Can you work these out from the model? Positions are in its coordinate system, mm. A direction names the side the tool comes from. Round coordinates to 2 decimals unless told otherwise and drop trailing zeros. Write each loop counter-clockwise with the first axis right and the second up, starting at its lowest first coordinate (ties: lowest second). Pieces come first, ordered by that corner, then holes. Notation, with made-up numbers: M 86.25,84.5 L 93.25,84.5 A5 cw 93.25,91.5 Z; hole C 24,31.25 d6. An arc over 180 degrees is marked long. Answer in a Markdown table with one row per item. Add a question column.
(1) I'm going to push flat-ended pins straight in: pin 1 (0.8 mm diameter, centred on x = -17.5, y = -6, fed in from +Z); pin 2 (4.5 mm diameter, centred on x = -12.5, z = 10.5, fed in from -Y); pin 3 (1.5 mm diameter, centred on y = -3, z = 11.5, fed in from +X). Where does each tip first touch, or does it pass through?
(2) For faces 1 (the face through (10, -6, 5)), 2 (the face through (23, 5.2, 5)), 3 (the face through (11.343, 18.021, 3.889)), 4 (the face through (13, 6, 8)), 5 (the face through (0, 14.6, 1)), which set-ups out of +Z, -Z, +X, -X, +Y, -Y let a thin tool reach every point of the face, with its end or its side?
(3) Suppose I cut it at C-C, the plane x = 4. Write out the boundary of the cut face in (y, z).
(4) If I drill on probe 1 along Y at (x, z) = (-13, 5.25); probe 2 along X at (y, z) = (-6.5, 10.25); probe 3 along Y at (x, z) = (19, 13.25), over which ranges is the centre line in solid material (lowest first)?
(5) Suppose I cut it at D-D, the plane y = -4.5. Write out the boundary of the cut face in (x, z), then the cut area to 3 significant figures.
(6) Suppose I cut it at B-B, the plane x = -8.5. Write out the boundary of the cut face in (y, z), then the cut area to 3 significant figures.
(7) If we mould it in two halves opening along X, with no side actions, what happens to faces 6 (the face through (-22.5, -12.5, 1.5)), 7 (the face through (0, -10.4, 1)), 8 (the face through (25, 0, 2)), 9 (the face through (-22, 17, 4))? For each: released by +X, released by -X, zero draft, split by the parting line, or undercut.
(8) Suppose I cut it at A-A, the plane y = -12.5. Write out the boundary of the cut face in (x, z), then the cut area to 3 significant figures.
from build123d import *

# Parameters (mm, degrees)
SZKIC1_W                    = 50
SZKIC1_H                    = 34
DODANIE_WYCI_GNI_CIE1_DEPTH = 3
WYTNIJ_WYCI_GNI_CIE1_DEPTH  = 31.380915062
SZKIC2_W                    = 50
SZKIC2_H                    = 1.3
SZKIC2_W_2                  = 15
SZKIC2_H_2                  = 1.6
DODANIE_WYCI_GNI_CIE2_DEPTH = 5
DODANIE_WYCI_GNI_CIE5_DEPTH = 8
SZKIC9_R                    = 0.85
WYTNIJ_WYCI_GNI_CIE3_DEPTH  = 3
WYTNIJ_WYCI_GNI_CIE4_DEPTH  = 1
SZKIC5_W                    = 4
SZKIC5_H                    = 13.6
DODANIE_WYCI_GNI_CIE3_DEPTH = 15
DODANIE_WYCI_GNI_CIE4_START = -6.8
DODANIE_WYCI_GNI_CIE4_DEPTH = 13.6
SZKIC7_R                    = 0.85
WYTNIJ_WYCI_GNI_CIE2_DEPTH  = 8


with BuildPart() as part:
    # Szkic1 → Dodanie-wyciągnięcie1 (new body)
    with BuildSketch(Plane.XY):
        Rectangle(SZKIC1_W, SZKIC1_H)
    extrude(amount=DODANIE_WYCI_GNI_CIE1_DEPTH)

    # Szkic3 → Wytnij-wyciągnięcie1 (cut, through all)
    with BuildSketch(Plane.XY):
        with BuildLine():
            Line((-20.4, 14.6), (20.4, 14.6))
            ThreePointArc((20.4, 14.6), (22.5, 12.5), (20.4, 10.4))
            Line((20.4, 10.4), (-20.4, 10.4))
            ThreePointArc((-20.4, 10.4), (-22.5, 12.5), (-20.4, 14.6))
        make_face()
    wytnij_wyci_gni_cie1 = extrude(amount=WYTNIJ_WYCI_GNI_CIE1_DEPTH, mode=Mode.SUBTRACT)

    # Szkic2 → Dodanie-wyciągnięcie2 (add)
    with BuildSketch(Plane.XY.offset(3)):
        with Locations((0, 16.35)):
            Rectangle(SZKIC2_W, SZKIC2_H)
        with Locations((-17.5, 6)):
            Rectangle(SZKIC2_W_2, SZKIC2_H_2)
        with Locations((17.5, 6)):
            Rectangle(SZKIC2_W_2, SZKIC2_H_2)
    dodanie_wyci_gni_cie2 = extrude(amount=DODANIE_WYCI_GNI_CIE2_DEPTH)

    # Lustro1: Wytnij-wyciągnięcie1, Dodanie-wyciągnięcie2 across plane
    add(wytnij_wyci_gni_cie1.mirror(Plane.ZX), mode=Mode.SUBTRACT)
    add(dodanie_wyci_gni_cie2.mirror(Plane.ZX))

    # Szkic8 → Dodanie-wyciągnięcie5 (add)
    with BuildSketch(Plane(origin=(0, 0, 0), x_dir=(-1, 0, 0), z_dir=(0, 0, -1))):
        Polygon((-18.5, 17), (-16, 19.5), (16, 19.5), (18.5, 17), align=None)
    extrude(amount=-DODANIE_WYCI_GNI_CIE5_DEPTH)

    # Szkic9 → Wytnij-wyciągnięcie3 (cut)
    with BuildSketch(Plane(origin=(0, 19.5, 0), x_dir=(1, 0, 0), z_dir=(0, 1, 0))):
        with Locations(Location((-10.5, -4, 0), (0, 0, 270))):
            Circle(SZKIC9_R)
        with Locations(Location((10.5, -4, 0), (0, 0, 270))):
            Circle(SZKIC9_R)
    extrude(amount=-WYTNIJ_WYCI_GNI_CIE3_DEPTH, mode=Mode.SUBTRACT)

    # Szkic9<3> → Wytnij-wyciągnięcie4 (cut)
    with BuildSketch(Plane(origin=(0, 19.5, 0), x_dir=(1, 0, 0), z_dir=(0, 1, 0))):
        with BuildLine():
            ThreePointArc((2.5, -4), (1.767766953, -2.232233047), (0, -1.5))
            Line((0, -1.5), (0, -6.5))
            ThreePointArc((0, -6.5), (1.767766953, -5.767766953), (2.5, -4))
        make_face()
        with BuildLine():
            Line((0, -6.5), (0, -1.5))
            ThreePointArc((0, -1.5), (-2.5, -4), (0, -6.5))
        make_face()
    extrude(amount=-WYTNIJ_WYCI_GNI_CIE4_DEPTH, mode=Mode.SUBTRACT)

    # Szkic5 → Dodanie-wyciągnięcie3 (add)
    with BuildSketch(Plane.XY.offset(3)):
        with Locations((19, 0)):
            Rectangle(SZKIC5_W, SZKIC5_H)
        with Locations((-12, 0)):
            Rectangle(SZKIC5_W, SZKIC5_H)
    extrude(amount=DODANIE_WYCI_GNI_CIE3_DEPTH)

    # Szkic6 → Dodanie-wyciągnięcie4 (add)
    with BuildSketch(Plane(origin=(0, 0, 0), x_dir=(1, 0, 0), z_dir=(0, 1, 0)).offset(DODANIE_WYCI_GNI_CIE4_START)):
        Polygon((-10, -18), (-6.5, -18), (-6.5, -14.5), (-10, -11), align=None)
    extrude(amount=DODANIE_WYCI_GNI_CIE4_DEPTH)

    # Szkic7 → Wytnij-wyciągnięcie2 (cut)
    with BuildSketch(Plane.XY.offset(18)):
        with Locations((-8.5, 0)):
            Circle(SZKIC7_R)
        with Locations((19, 0)):
            Circle(SZKIC7_R)
    extrude(amount=-WYTNIJ_WYCI_GNI_CIE2_DEPTH, mode=Mode.SUBTRACT)


solid = part.part
Calculated:
| question | item | result |
|---|---|---|
| 1 | pin 1 | z = 8 |
| 1 | pin 2 | y = -6.8 |
| 1 | pin 3 | x = 21 |
| 2 | face 1 | +Z |
| 2 | face 2 | +Z, +X |
| 2 | face 3 | +Y |
| 2 | face 4 | +Z, +Y, -Y |
| 2 | face 5 | +Z, -Z |
| 3 | outline | M -17,0 L -14.6,0 L -14.6,3 L -15.7,3 L -15.7,8 L -17,8 Z; M -10.4,0 L 10.4,0 L 10.4,3 L -10.4,3 Z; M 14.6,0 L 19.5,0 L 19.5,8 L 15.7,8 L 15.7,3 L 14.6,3 Z |
| 4 | probe 1 | -17 to -15.7, -6.8 to 6.8, 15.7 to 19.5 |
| 4 | probe 2 | -14 to -10, 17 to 21 |
| 4 | probe 3 | -6.8 to -0.85, 0.85 to 6.8 |
| 5 | outline | M -25,0 L 25,0 L 25,3 L 21,3 L 21,18 L 17,18 L 17,3 L -10,3 L -10,11 L -6.5,14.5 L -6.5,18 L -14,18 L -14,3 L -25,3 Z |
| 5 | area | 288 mm² |
| 6 | outline | M -17,0 L -14.6,0 L -14.6,3 L -15.7,3 L -15.7,8 L -17,8 Z; M -10.4,0 L 10.4,0 L 10.4,3 L -10.4,3 Z; M -6.8,12.5 L -0.85,12.5 L -0.85,18 L -6.8,18 Z; M 0.85,12.5 L 6.8,12.5 L 6.8,18 L 0.85,18 Z; M 14.6,0 L 19.5,0 L 19.5,8 L 15.7,8 L 15.7,3 L 14.6,3 Z |
| 6 | area | 175 mm² |
| 7 | face 6 | undercut |
| 7 | face 7 | undercut |
| 7 | face 8 | released by +X |
| 7 | face 9 | zero draft |
| 8 | outline | M -25,0 L -22.5,0 L -22.5,3 L -25,3 Z; M 22.5,0 L 25,0 L 25,3 L 22.5,3 Z |
| 8 | area | 15.0 mm² |
